Design review of the part built by this model. Coordinates are the model's own, in mm. A direction names the side the tool comes from. Coordinates: 2 decimals unless noted, no trailing zeros. Loops run counter-clockwise (first coordinate to the right, second up) from the corner with the lowest first, then second, coordinate; pieces in that order, holes last. Notation, with made-up numbers: (-15.5, -6.75) -> (7.5, -6.75) arc R20 cw to (7.5, 10.25) -> close; hole circle Ø5 at (-39.75, 1). An arc over 180 degrees is marked (long way). Use CSV: the item, a comma, the result in double quotes.
```python
from build123d import *

# Parameters (mm, degrees)
SKETCH_2_R          = 2.5
CUT_EXTRUDE_3_DEPTH = 20
EXTRUDE_START       = 20
SKETCH_4_R          = 3
SKETCH_4_R_2        = 2.5
EXTRUDE_1_DEPTH     = 20
SKETCH_5_W          = 2.680740698
SKETCH_5_H          = 11
EXTRUDE_2_DEPTH     = 50


with BuildPart() as part:
    # 草圖1 → 旋轉2 (revolve)
    with BuildSketch(Plane.XY, mode=Mode.PRIVATE) as revolve_2_sk:
        Polygon((0, 8.5), (0, 0), (12, 0), align=None)
    revolve(revolve_2_sk.sketch.rotate(Axis((0, 0, 0), (1, 0, 0)), 90), axis=Axis((0, 0, 0), (1, 0, 0)))

    # 草圖2 → 除料-伸長3 (cut)
    with BuildSketch(Plane.ZY):
        Circle(SKETCH_2_R)
    extrude(amount=-CUT_EXTRUDE_3_DEPTH, mode=Mode.SUBTRACT)

    # 草圖4 → 填料-伸長1 (add)
    with BuildSketch(Plane.ZY.offset(EXTRUDE_START)):
        with Locations(Location((0, 0, 0), (0, 0, 180))):
            Circle(SKETCH_4_R)
        Circle(SKETCH_4_R_2, mode=Mode.SUBTRACT)
    extrude(amount=-EXTRUDE_1_DEPTH)

    # 草圖5 → 填料-伸長2 (add)
    with BuildSketch(Plane.ZY):
        with Locations((-5.140370349, 0)):
            Rectangle(SKETCH_5_W, SKETCH_5_H)
    extrude(amount=EXTRUDE_2_DEPTH)


solid = part.part
```
Item 1: Add section D-D (x = -43). Give the boundary of the cut face in (y, z).
Checked values:
outline,"(-5.5, -6.48) -> (5.5, -6.48) -> (5.5, -3.8) -> (-5.5, -3.8) -> close"
Item 2: Machinability: for faces 4 (the face through (-25, 0, -3.8)), 5 (the face through (-20, -2, 2)), 6 (the face through (0, 0, -7)), which of the approach directions +Z, -Z, +X, -X, +Y, -Y give a long, thin tool a straight path to every point of the face, cutting with its end or side? Answer none if there is none.
Checked values:
face 4,"-X, +Y, -Y"
face 5,"+Z, -X, +Y, -Y"
face 6,"-Z, -X, +Y, -Y"
Item 3: Clearance check with flat-ended pins moving along their axes: pin 1 (5 mm diameter, centred on y = 0.5, z = 0.5, fed in from -X); pin 2 (2 mm diameter, centred on x = -1.5, y = -6, fed in from +Z); pin 3 (1.5 mm diameter, centred on y = -2.5, z = -6.5, fed in from +X). State where each tip first meets the part, or that it passes through.
Checked values:
pin 1,"x = -20"
pin 2,"z = -3.8"
pin 3,"x = 3.23"
Item 4: Add section B-B (y = 0). Give the boundary of the cut face in (x, z).
Checked values:
outline,"(-50, -6.48) -> (0, -6.48) -> (0, -8.5) -> (8.47, -2.5) -> (-20, -2.5) -> (-20, -3) -> (0, -3) -> (0, -3.8) -> (-50, -3.8) -> close; (-20, 2.5) -> (8.47, 2.5) -> (0, 8.5) -> (0, 3) -> (-20, 3) -> close"
Item 5: Draft analysis for pull direction Z (two halves, no side actions). For faces 1 (the face through (-5.96, -2.44, -0.54)), 2 (the face through (-25, 5.5, -5)), 3 (the face through (7, 2.155, -2.811)), state which applies: pulls with the +Z half, pulls with the -Z half, needs draft (parallel to the pull), parting line crosses it, or undercut.
Checked values:
face 1,"undercut"
face 2,"needs draft"
face 3,"parting line crosses it"
Item 6: Add section C-C (z = 0). Give the boundary of the cut face in (x, y), then the cut area to 3 significant figures.
Checked values:
outline,"(-20, -3) -> (0, -3) -> (0, -8.5) -> (8.47, -2.5) -> (-20, -2.5) -> close; (-20, 2.5) -> (8.47, 2.5) -> (0, 8.5) -> (0, 3) -> (-20, 3) -> close"
area,"70.8 mm^2"
Item 7: Add section A-A (x = -8). Give the boundary of the cut face in (y, z).
Checked values:
outline,"(-5.5, -6.48) -> (5.5, -6.48) -> (5.5, -3.8) -> (-5.5, -3.8) -> close; circle Ø6 at (0, 0); hole circle Ø5 at (0, 0)"
Item 8: To check wall thickness, follow line 1 along Y through (x, z) = (-7.75, 0); line 2 along Y through (x, z) = (-27, -5.75); line 3 along Z through (x, y) = (-25.5, 5). State the ranges of each line that lie inside material, in increasing order.
Checked values:
line 1,"-3 to -2.5, 2.5 to 3"
line 2,"-5.5 to 5.5"
line 3,"-6.48 to -3.8"
